For this review, use the dimensioned drawing (mm, ordinates from the lowest corner) and the shaded views. Round coordinates to 2 decimals unless told otherwise and drop trailing zeros. Write each loop counter-clockwise with the first axis right and the second up, starting at its lowest first coordinate (ties: lowest second). Pieces come first, ordered by that corner, then holes.
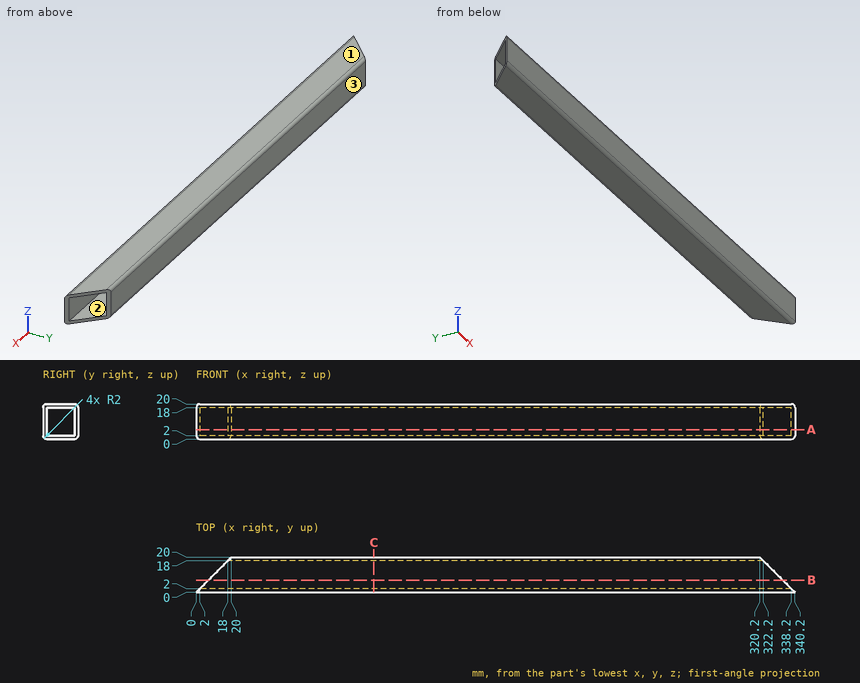
(1) For line 1 along Z through (x, y) = (210.5, 8); line 2 along Y through (x, z) = (322, 9.5), list the stretches that pass through material, from the lowest coordinate up.
Geometry check:
line 1: z = 0 to 2, 18 to 20
line 2: y = 0 to 2, 18 to 18.2
(2) For pin 1 Ø4 at (x, y) = (196.5, 12) entering from -Z; pin 2 Ø12 at (y, z) = (14.5, 17.5) entering from -X, all flat-tipped, find the tip position at first contact; note any pin that passes through.
Geometry check:
pin 1: stops at z = 0
pin 2: stops at x = 8.52
(3) Mouldability with a two-part tool opening along Y and no side actions: class the marked faces 1, 2 and 3 as pulls with the +Y half, pulls with the -Y half, needs draft (parallel to the pull), parting line crosses it, or undercut.
Geometry check:
face 1: needs draft
face 2: undercut
face 3: pulls with the +Y half
(4) We need section A-A, the plane z = 5.5. Give the boundary of the cut face in (x, y), and give its area (3 significant figures).
Geometry check:
outline: (0, 0) - (340.2, 0) - (338.2, 2) - (2, 2) - close; (18, 18) - (322.2, 18) - (320.2, 20) - (20, 20) - close
area: 1,280 mm2
(5) We need section C-C, the plane x = 101. Give the boundary of the cut face in (y, z), and give its area (3 significant figures).
Geometry check:
outline: (0, 2) arc R2 ccw to (2, 0) - (18, 0) arc R2 ccw to (20, 2) - (20, 18) arc R2 ccw to (18, 20) - (2, 20) arc R2 ccw to (0, 18) - close; hole (2, 2) - (18, 2) - (18, 18) - (2, 18) - close
area: 141 mm2
(6) We need section B-B, the plane y = 7. Give the boundary of the cut face in (x, z).
Geometry check:
outline: (7, 0) - (333.2, 0) - (333.2, 2) - (7, 2) - close; (7, 18) - (333.2, 18) - (333.2, 20) - (7, 20) - close
